Work out the finished part from the listing and answer in its coordinate system (mm). Coordinates: 2 decimals unless noted, no trailing zeros. Write each loop counter-clockwise with the first axis right and the second up, starting at its lowest first coordinate (ties: lowest second). Pieces come first, ordered by that corner, then holes. Notation, with made-up numbers: (-0.75, 38) - (41.25, 38) arc R14 ccw to (41.25, 51) - close; hole circle Ø3 at (-0.75, 3). An arc over 180 degrees is marked (long way). One line per item, written item: value.
```python
from build123d import *

# Parameters (mm, degrees)
F1_DEPTH = 5
F3_DEPTH = 25


with BuildPart() as f1:
    # F0 (on Top) → F1 (new body)
    with BuildSketch(Plane.XY):
        with BuildLine():
            Line((145, -225), (173, -225))
            ThreePointArc((173, -225), (174.4142135624, -224.4142135624), (175, -223))
            Line((175, -223), (175, 223))
            ThreePointArc((175, 223), (174.4142135624, 224.4142135624), (173, 225))
            Line((173, 225), (145, 225))
            Line((145, 225), (145, 230))
            Line((145, 230), (160, 230))
            Line((160, 230), (160, 238))
            ThreePointArc((160, 238), (159.4142135624, 239.4142135624), (158, 240))
            Line((158, 240), (62, 240))
            ThreePointArc((62, 240), (60.5857864376, 239.4142135624), (60, 238))
            Line((60, 238), (60, 230))
            Line((60, 230), (-123, 230))
            ThreePointArc((-123, 230), (-124.4142135624, 229.4142135624), (-125, 228))
            Line((-125, 228), (-125, 227))
            ThreePointArc((-125, 227), (-125.5857864376, 225.5857864376), (-127, 225))
            Line((-127, 225), (-173, 225))
            ThreePointArc((-173, 225), (-174.4142135624, 224.4142135624), (-175, 223))
            Line((-175, 223), (-175, -223))
            ThreePointArc((-175, -223), (-174.4142135624, -224.4142135624), (-173, -225))
            Line((-173, -225), (-127, -225))
            ThreePointArc((-127, -225), (-125.5857864376, -225.5857864376), (-125, -227))
            Line((-125, -227), (-125, -228))
            ThreePointArc((-125, -228), (-124.4142135624, -229.4142135624), (-123, -230))
            Line((-123, -230), (58, -230))
            ThreePointArc((58, -230), (59.4142135624, -230.5857864376), (60, -232))
            Line((60, -232), (60, -238))
            ThreePointArc((60, -238), (60.5857864376, -239.4142135624), (62, -240))
            Line((62, -240), (158, -240))
            ThreePointArc((158, -240), (159.4142135624, -239.4142135624), (160, -238))
            Line((160, -238), (160, -230))
            Line((160, -230), (145, -230))
            Line((145, -230), (145, -225))
        make_face()
    extrude(amount=F1_DEPTH)

    # F2 (on face) → F3 (cut)
    with BuildSketch(Plane.XY.offset(5)):
        with BuildLine():
            Line((-161, 225), (-161, 340.5782580579))
            Line((-161, 340.5782580579), (-227.952612991, 340.5782580579))
            Line((-227.952612991, 340.5782580579), (-227.952612991, -338.3395225013))
            Line((-227.952612991, -338.3395225013), (-161, -338.3395225013))
            Line((-161, -338.3395225013), (-161, -225))
            Line((-161, -225), (-173, -225))
            ThreePointArc((-173, -225), (-174.4142135624, -224.4142135624), (-175, -223))
            Line((-175, -223), (-175, 223))
            ThreePointArc((-175, 223), (-174.4142135624, 224.4142135624), (-173, 225))
            Line((-173, 225), (-161, 225))
        make_face()
        with BuildLine():
            Line((-161, -225), (-161, 225))
            Line((-161, 225), (-173, 225))
            ThreePointArc((-173, 225), (-174.4142135624, 224.4142135624), (-175, 223))
            Line((-175, 223), (-175, -223))
            ThreePointArc((-175, -223), (-174.4142135624, -224.4142135624), (-173, -225))
            Line((-173, -225), (-161, -225))
        make_face()
    extrude(amount=-F3_DEPTH, mode=Mode.SUBTRACT)


solid = f1.part
```
Item 1: Section B-B, the plane x = -84 is taken. Determine the outline of the cut face in (y, z).
Evaluation:
outline: (-230, 0) - (230, 0) - (230, 5) - (-230, 5) - close
Item 2: Given pin 1 (1.5 mm diameter, centred on x = -47, z = 4.5, fed in from -Y); pin 2 (1.5 mm diameter, centred on x = 33, y = 166, fed in from -Z); pin 3 (2.5 mm diameter, centred on y = -226.5, z = 3.5, fed in from +X); pin 4 (1.5 mm diameter, centred on y = -232.5, z = 2, fed in from +X), each flat-ended and moving along its own axis, determine where each tip first touches the part or whether it passes through.
Evaluation:
pin 1: stops at y = -230
pin 2: stops at z = 0
pin 3: stops at x = 145
pin 4: stops at x = 160
Item 3: Consider probe 1 along Y at (x, z) = (-73.5, 0.45); probe 2 along Y at (x, z) = (-134.5, 1.75). Determine where each line is inside the solid, lowest interval first.
Evaluation:
probe 1: y = -230 to 230
probe 2: y = -225 to 225
